Can you work these out from the model? Positions are in its coordinate system, mm. Coordinates: 2 decimals unless noted, no trailing zeros. Order: outer loops, then holes, each group sorted by start corner. A loop starts at its lowest first (then second) coordinate and runs counter-clockwise, first axis right, second up. Notation, with made-up numbers: (58.5, -9.5) -> (95.5, -9.5) arc R21 cw to (95.5, 21.5) -> close; hole circle Ø6 at (-29, 37). An arc over 180 degrees is marked (long way). Return JSON: item names as keys, results as strings. Group by question number.
1) Thinking about a two-plate mould opening in Z: for faces 1 (the cylindrical face through (-1.5, 0.07, 18.93)), 2 (the flat face through (0, 0, -1)), 3 (the flat face through (0, 0, 38.5)), 4 (the cylindrical face through (-0.17, 1.29, -0.25)), which applies, +Z half, -Z half, draft (parallel to the pull), parting line (faces both ways), or undercut?
2) If we section it at A-A, the plane z = 34.5: Please give me the cut outline in (x, y).
3) If I drill on probe 1 along Y at (x, z) = (0.55, 24.5); probe 2 along Y at (x, z) = (0.15, 24); probe 3 along X at (y, z) = (0.7, 5), over which ranges is the centre line in solid material (lowest first)? Write a range as from..to.
from build123d import *

# Parameters (mm, degrees)
F0_R     = 1.5
F0_R_2   = 1.3
F1_DEPTH = 38.5
F2_DEPTH = 1
F3_START = -0.5
F3_DEPTH = 0.5
F4_SIZE  = 0.2
F5_SIZE  = 0.1


with BuildPart() as f1:
    # F0 (on Top) → F1 (new body)
    with BuildSketch(Plane.XY):
        Circle(F0_R)
        Circle(F0_R_2, mode=Mode.SUBTRACT)
        Circle(F0_R_2)
    extrude(amount=F1_DEPTH)

    # F0 (on Top) → F2 (join)
    with BuildSketch(Plane.XY):
        Circle(F0_R_2)
    extrude(amount=-F2_DEPTH)

    # F0 (on Top) → F3 (join)
    with BuildSketch(Plane.XY.offset(F3_START)):
        Circle(F0_R)
        Circle(F0_R_2, mode=Mode.SUBTRACT)
    extrude(amount=-F3_DEPTH)

    # F4
    f4_edges = [f1.edges().sort_by_distance(p)[0] for p in [
        (-1.5, 0, -1),
        (-1.5, 0, 38.5),
    ]]
    chamfer(f4_edges, length=F4_SIZE)

    # F5
    f5_edges = [f1.edges().sort_by_distance(p)[0] for p in [
        (-1.5, 0, -0.5),
        (-1.5, 0, 0),
    ]]
    chamfer(f5_edges, length=F5_SIZE)


solid = f1.part
Result sheet:
{
 "1": {"face 1": "draft", "face 2": "-Z half", "face 3": "+Z half", "face 4": "undercut"},
 "2": {"outline": "circle Ø3 at (0, 0)"},
 "3": {"probe 1": "y = -1.4..1.4", "probe 2": "y = -1.49..1.49", "probe 3": "x = -1.33..1.33"}
}
